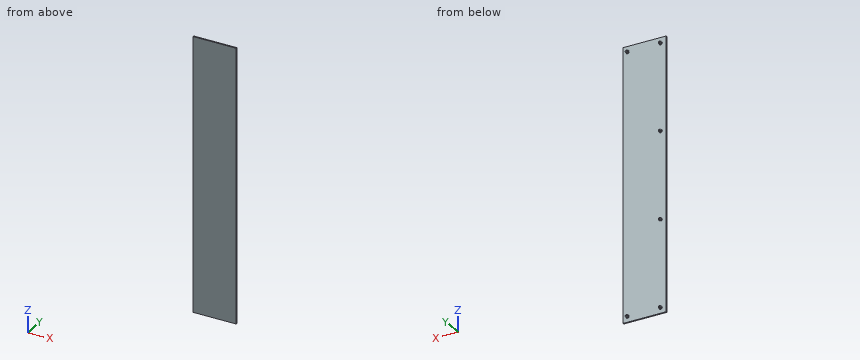
Autodesk Inventor part; units mm, degrees
ref_plane "YZ Plane" through (0, 0, 0) normal (1, 0, 0) x (0, 1, 0)
ref_plane "XZ Plane" through (0, 0, 0) normal (0, 1, 0) x (-1, 0, 0)
ref_plane "XY Plane" through (0, 0, 0) normal (0, 0, 1) x (1, 0, 0)
sketch "Esboço1" plane through (0, 0, 0) normal (0, 1, 0) x (-1, 0, 0)
  line L0 (0, 0) -> (-100.5, 0)
  line L1 (-100.5, 0) -> (-100.5, -640.37)
  line L2 (-100.5, -640.37) -> (0, -640.37)
  line L3 (0, -640.37) -> (0, 0)
  dimension "d0" = 100.5
  dimension "d1" = 640.37
extrude "Extrusão1" add sketch "Esboço1" along normal blind 3
sketch "Esboço2" plane through (0, 3, 0) normal (0, 1, 0) x (1, 0, 0)
  line L0 (0, 0) -> (100.5, 0)
  line L1 (0, 0) -> (100.5, 0)
  line L2 (0, 20) -> (0, 0)
  line L3 (100.5, 640.37) -> (0, 640.37)
  line L4 (0, 0) -> (23, 0)
  line L5 (23, 0) -> (23, 640.37)
  line L6 (23, 640.37) -> (0, 640.37)
  line L7 (0, 640.37) -> (0, 0)
  line L8 (0, 640.37) -> (3, 640.37)
  line L9 (3, 640.37) -> (3, 0)
  line L10 (3, 0) -> (0, 0)
  line L11 (0, 0) -> (0, 640.37)
  line L12 (100.5, 0) -> (100.5, 640.37)
  line L13 (0, 0) -> (100.5, 0)
  line L14 (100.5, 0) -> (100.5, 23)
  line L15 (100.5, 23) -> (0, 23)
  line L16 (0, 23) -> (0, 0)
  line L17 (0, 23) -> (100.5, 23)
  line L18 (100.5, 23) -> (100.5, 3)
  line L19 (100.5, 3) -> (0, 3)
  line L20 (0, 3) -> (0, 23)
  line L21 (0, 640.37) -> (100.5, 640.37)
  line L22 (100.5, 640.37) -> (100.5, 617.37)
  line L23 (100.5, 617.37) -> (0, 617.37)
  line L24 (0, 617.37) -> (0, 640.37)
  line L25 (0, 617.37) -> (100.5, 617.37)
  line L26 (100.5, 617.37) -> (100.5, 637.37)
  line L27 (100.5, 637.37) -> (0, 637.37)
  line L28 (0, 637.37) -> (0, 617.37)
  line L29 (3, 617.37) -> (13, 617.37)
  line L30 (13, 617.37) -> (13, 627.37)
  line L31 (13, 627.37) -> (3, 627.37)
  line L32 (3, 627.37) -> (3, 617.37)
  line L33 (100.5, 617.37) -> (90.5, 617.37)
  line L34 (90.5, 617.37) -> (90.5, 627.37)
  line L35 (90.5, 627.37) -> (100.5, 627.37)
  line L36 (100.5, 627.37) -> (100.5, 617.37)
  line L37 (0, 320.185) -> (42.8938, 320.185)
  line L38 (0, 320.185) -> (13, 320.185)
  circle A0 centre (13, 320.185) radius 3
  circle A1 centre (13, 627.37) radius 3
  circle A2 centre (90.5, 627.37) radius 3
  line L39 (13, 320.185) -> (13, 422.58)
  line L40 (13, 422.58) -> (13, 524.975)
  circle A3 centre (13, 422.58) radius 3
  circle A4 centre (13, 524.975) radius 3
  circle A5 centre (13, 320.185) radius 3
  circle A6 centre (13, 13) radius 3
  circle A7 centre (90.5, 13) radius 3
  circle A8 centre (13, 217.79) radius 3
  circle A9 centre (13, 115.395) radius 3
  dimension "d5" = 23
  dimension "d6" = 3
  dimension "d7" = 23
  dimension "d8" = 20
  dimension "d9" = 23
  dimension "d10" = 20
  dimension "d11" = 10
  dimension "d12" = 10
  dimension "d13" = 10
  dimension "d14" = 6
  dimension "d15" = 6
  dimension "d16" = 6
  dimension "d17" = 102.395
  dimension "d18" = 102.395
extrude "Extrusão2" add sketch "Esboço2" along normal blind 4 contours A4 | A3 L40 L39 | L39 L40 A3 | A0 L39 L37 | L37 A0 | L37 L39 A0 | A1 L30 L31 | L31 L30 A1 | A2 L34 L35 | L35 L34 A2 | A6 | A7 | A8 | A9
sketch "Esboço3" plane through (0, 3, 0) normal (0, 1, 0) x (1, 0, 0)
  circle A0 centre (13, 13) radius 3
  circle A1 centre (13, 13) radius 4
  circle A2 centre (90.5, 13) radius 3
  circle A3 centre (90.5, 13) radius 4
  circle A4 centre (13, 115.395) radius 3
  circle A5 centre (13, 115.395) radius 4
  circle A6 centre (13, 217.79) radius 3
  circle A7 centre (13, 217.79) radius 4
  circle A8 centre (13, 320.185) radius 3
  circle A9 centre (13, 320.185) radius 4
  line L0 (100.5, 0) -> (100.5, 640.37)
  line L1 (100.5, 320.185) -> (82.1081, 320.185)
  circle A10 centre (13, 627.37) radius 3
  circle A11 centre (13, 627.37) radius 4
  circle A12 centre (90.5, 627.37) radius 3
  circle A13 centre (90.5, 627.37) radius 4
  circle A14 centre (13, 524.975) radius 3
  circle A15 centre (13, 524.975) radius 4
  circle A16 centre (13, 422.58) radius 3
  circle A17 centre (13, 422.58) radius 4
  circle A18 centre (13, 320.185) radius 3
  circle A19 centre (13, 320.185) radius 4
  point P0 (0, 0)
  dimension "d21" = 8
  dimension "d22" = 8
  dimension "d23" = 8
  dimension "d24" = 8
  dimension "d25" = 8
extrude "Extrusão3" add sketch "Esboço3" along normal blind 1 contours A0 | A1 | A2 | A3 | A4 | A5 | A6 | A7 | A8 | A9 | A10 | A11 | A12 | A13 | A14 | A15 | A16 | A17
sketch "Esboço4" plane through (13, 7, -13) normal (0, 1, 0) x (1, 0, 0)
  circle A0 centre (0, 0) radius 3
  line L0 (0, 0) -> (1.5, 0)
  circle A1 centre (0, 0) radius 4
  line L1 (1.5, 0) -> (0.75, -1.299)
  line L2 (0.75, -1.299) -> (-0.75, -1.299)
  line L3 (-0.75, -1.299) -> (-1.5, 0)
  line L4 (-1.5, 0) -> (-0.75, 1.299)
  line L5 (-0.75, 1.299) -> (0.75, 1.299)
  line L6 (0.75, 1.299) -> (1.5, 0)
  circle A2 centre (77.5, 0) radius 3
  line L7 (77.5, 0) -> (79, 0)
  line L8 (79, 0) -> (78.25, -1.299)
  line L9 (78.25, -1.299) -> (76.75, -1.299)
  line L10 (76.75, -1.299) -> (76, 0)
  line L11 (76, 0) -> (76.75, 1.299)
  line L12 (76.75, 1.299) -> (78.25, 1.299)
  line L13 (78.25, 1.299) -> (79, 0)
  circle A3 centre (0, 102.395) radius 3
  line L14 (0, 102.395) -> (1.5, 102.395)
  line L15 (1.5, 102.395) -> (0.75, 101.096)
  line L16 (0.75, 101.096) -> (-0.75, 101.096)
  line L17 (-0.75, 101.096) -> (-1.5, 102.395)
  line L18 (-1.5, 102.395) -> (-0.75, 103.694)
  line L19 (-0.75, 103.694) -> (0.75, 103.694)
  line L20 (0.75, 103.694) -> (1.5, 102.395)
  circle A4 centre (0, 204.79) radius 3
  line L21 (0, 204.79) -> (1.5, 204.79)
  line L22 (1.5, 204.79) -> (0.75, 203.491)
  line L23 (0.75, 203.491) -> (-0.75, 203.491)
  line L24 (-0.75, 203.491) -> (-1.5, 204.79)
  line L25 (-1.5, 204.79) -> (-0.75, 206.089)
  line L26 (-0.75, 206.089) -> (0.75, 206.089)
  line L27 (0.75, 206.089) -> (1.5, 204.79)
  circle A5 centre (0, 307.185) radius 4
  line L28 (0, 307.185) -> (1.5, 307.185)
  circle A6 centre (0, 307.185) radius 3
  line L29 (1.5, 307.185) -> (0.75, 305.886)
  line L30 (0.75, 305.886) -> (-0.75, 305.886)
  line L31 (-0.75, 305.886) -> (-1.5, 307.185)
  line L32 (-1.5, 307.185) -> (-0.75, 308.484)
  line L33 (-0.75, 308.484) -> (0.75, 308.484)
  line L34 (0.75, 308.484) -> (1.5, 307.185)
  line L35 (87.5, -13) -> (87.5, 627.37)
  line L36 (87.5, 307.185) -> (57.6178, 307.185)
  circle A7 centre (0, 614.37) radius 3
  line L37 (0, 614.37) -> (1.5, 614.37)
  circle A8 centre (0, 614.37) radius 4
  line L38 (1.5, 614.37) -> (0.75, 615.669)
  line L39 (0.75, 615.669) -> (-0.75, 615.669)
  line L40 (-0.75, 615.669) -> (-1.5, 614.37)
  line L41 (-1.5, 614.37) -> (-0.75, 613.071)
  line L42 (-0.75, 613.071) -> (0.75, 613.071)
  line L43 (0.75, 613.071) -> (1.5, 614.37)
  circle A9 centre (77.5, 614.37) radius 3
  line L44 (77.5, 614.37) -> (79, 614.37)
  line L45 (79, 614.37) -> (78.25, 615.669)
  line L46 (78.25, 615.669) -> (76.75, 615.669)
  line L47 (76.75, 615.669) -> (76, 614.37)
  line L48 (76, 614.37) -> (76.75, 613.071)
  line L49 (76.75, 613.071) -> (78.25, 613.071)
  line L50 (78.25, 613.071) -> (79, 614.37)
  circle A10 centre (0, 511.975) radius 3
  line L51 (0, 511.975) -> (1.5, 511.975)
  line L52 (1.5, 511.975) -> (0.75, 513.274)
  line L53 (0.75, 513.274) -> (-0.75, 513.274)
  line L54 (-0.75, 513.274) -> (-1.5, 511.975)
  line L55 (-1.5, 511.975) -> (-0.75, 510.676)
  line L56 (-0.75, 510.676) -> (0.75, 510.676)
  line L57 (0.75, 510.676) -> (1.5, 511.975)
  circle A11 centre (0, 409.58) radius 3
  line L58 (0, 409.58) -> (1.5, 409.58)
  line L59 (1.5, 409.58) -> (0.75, 410.879)
  line L60 (0.75, 410.879) -> (-0.75, 410.879)
  line L61 (-0.75, 410.879) -> (-1.5, 409.58)
  line L62 (-1.5, 409.58) -> (-0.75, 408.281)
  line L63 (-0.75, 408.281) -> (0.75, 408.281)
  line L64 (0.75, 408.281) -> (1.5, 409.58)
  circle A12 centre (0, 307.185) radius 4
  circle A13 centre (0, 307.185) radius 3
  line L65 (1.5, 307.185) -> (0.75, 308.484)
  line L66 (0.75, 308.484) -> (-0.75, 308.484)
  line L67 (-0.75, 308.484) -> (-1.5, 307.185)
  line L68 (-1.5, 307.185) -> (-0.75, 305.886)
  line L69 (-0.75, 305.886) -> (0.75, 305.886)
  line L70 (0.75, 305.886) -> (1.5, 307.185)
  point P0 (-13, -13)
  dimension "d28" = 1.5
  dimension "d29" = 1.5
  dimension "d30" = 1.5
extrude "Extrusão4" cut sketch "Esboço4" against normal blind 1.5 contours L1 L2 L3 L4 L5 L6 | L8 L9 L10 L11 L12 L13 | L15 L16 L17 L18 L19 L20 | L22 L23 L24 L25 L26 L27 | L29 L30 L31 L32 L33 L34 | L43 L42 L41 L40 L39 L38 | L50 L49 L48 L47 L46 L45 | L57 L56 L55 L54 L53 L52 | L64 L63 L62 L61 L60 L59
sketch "Esboço5" plane through (0, 3, 0) normal (0, 1, 0) x (1, 0, 0)
  line L0 (4.5679, 103.4306) -> (23.4921, 103.4306)
  line L1 (23.4921, 103.4306) -> (23.4921, 130.838)
  line L2 (23.4921, 130.838) -> (4.5679, 130.838)
  line L3 (4.5679, 130.838) -> (4.5679, 103.4306)
  line L4 (4.5679, 310.9443) -> (23.4921, 310.9443)
  line L5 (23.4921, 310.9443) -> (23.4921, 337.6992)
  line L6 (23.4921, 337.6992) -> (4.5679, 337.6992)
  line L7 (4.5679, 337.6992) -> (4.5679, 310.9443)
  line L8 (4.5679, 512.5849) -> (23.4921, 512.5849)
  line L9 (23.4921, 512.5849) -> (23.4921, 537.3821)
  line L10 (23.4921, 537.3821) -> (4.5679, 537.3821)
  line L11 (4.5679, 537.3821) -> (4.5679, 512.5849)
  point P0 (0, 0)
extrude "Extrusão5" cut sketch "Esboço5" along normal blind 5
properties part number "chapa_frente_esquerda"
Source: CAD feature listing. Evaluate the final solid. Frame: model axes, mm. Round coordinates to 2 decimals unless told otherwise and drop trailing zeros. Order: outer loops, then holes, each group sorted by start corner. A loop starts at its lowest first (then second) coordinate and runs counter-clockwise, first axis right, second up. Notation, with made-up numbers: (1, 22.25) -> (54, 22.25) arc R22 cw to (54, 51.25) -> close; hole circle Ø1 at (-10, 81.25). An arc over 180 degrees is marked (long way). Answer as CSV lines item,"result".
Item 1: Line query: L1, parallel to Z at x = 13.5, y = 3.5; L2, parallel to Y at x = 96, z = -349.5. Output: solid intervals per line, ascending.
A:
L1,"-631.34 to -623.4, -426.55 to -418.61, -221.76 to -213.82, -16.97 to -9.03"
L2,"0 to 3"
Item 2: Section A-A, the plane z = -98. Return loops of the section in (x, y).
A:
outline,"(0, 0) -> (100.5, 0) -> (100.5, 3) -> (0, 3) -> close"
Item 3: Section B-B, the plane x = 25. Return loops of the section in (y, z), plus the area to 3 significant figures.
A:
outline,"(0, -640.37) -> (3, -640.37) -> (3, 0) -> (0, 0) -> close"
area,"1,920 mm²"
Item 4: Pin query (flat end, axial travel): pin 1 Ø1.6 at (x, y) = (90, 6) entering from +Z; pin 2 Ø1.2 at (x, y) = (90.5, 6) entering from -Z; pin 3 Ø0.8 at (x, z) = (91, -627.5) entering from +Y. Return the tip coordinate at first contact, or that it passes through.
A:
pin 1,"z = -10"
pin 2,"z = -630.37"
pin 3,"y = 5.5"
